Input: dimensioned drawing with shaded views. Units: mm. Origin: part minimum x, y, z. Give positions to 0.01 mm unless a question says otherwise; leave off trailing zeros. Loops run counter-clockwise (first coordinate to the right, second up) from the corner with the lowest first, then second, coordinate; pieces in that order, holes last. Notation, with made-up numbers: (59.5, 57) -> (107.5, 57) arc R30 ccw to (107.5, 94) -> close; hole circle Ø10 at (-5.75, -0.75). An arc over 180 degrees is marked (long way). Answer in a Markdown table with one row per item. Add a question column.
1) Line query: line 1 (Z direction, x = 59.5, y = 5.25); line 2 (Z direction, x = 4, y = 2.75) (1 decimal). Output: solid intervals per line, ascending. Write a range as from..to.
2) Section query C-C (z = 1). Return the cut outline in (x, y).
3) Draft query along X for the marked faces 1, 2 and 3. Return one class per face: +X half, -X half, draft (parallel to the pull), parting line (faces both ways), or undercut.
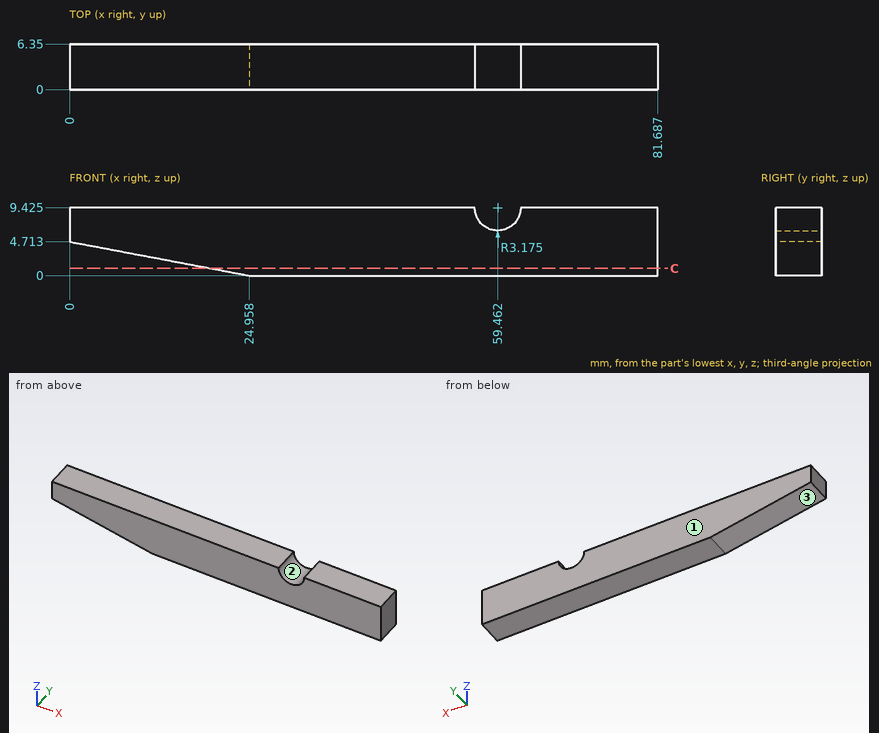
Evaluation:
| question | item | result |
|---|---|---|
| 1 | line 1 | 0..6.25 |
| 1 | line 2 | 4..9.4 |
| 2 | outline | (19.66, 0) -> (81.69, 0) -> (81.69, 6.35) -> (19.66, 6.35) -> close |
| 3 | face 1 | draft |
| 3 | face 2 | undercut |
| 3 | face 3 | -X half |
